Geometry: final body of the model. Coordinates: model frame, mm. Give positions to 0.01 mm unless a question says otherwise; leave off trailing zeros. Write each loop counter-clockwise with the first axis right and the second up, starting at its lowest first coordinate (ties: lowest second). Pieces come first, ordered by that corner, then holes. Notation, with made-up numbers: (-24, -16.5) - (4, -16.5) arc R20 cw to (4, 12.5) - close; hole circle Ø6 at (15, -3.75). An arc over 180 degrees is marked (long way). Use CSV: the item, a comma, the result in double quotes. Start each with the question number.
(1) First-contact query: pin 1 Ø1 at (y, z) = (5.5, -2) entering from -X; pin 2 Ø4 at (y, z) = (9, -1.5) entering from +X; pin 3 Ø1.5 at (y, z) = (26.5, 0.5) entering from -X. Flat tips, straight axial feed; report the tip coordinate or a pass-through.
(2) Section B-B on y = 13. Output: boundary loops of the cut face in (x, z), and give its area (3 significant figures).
(3) Section A-A on y = 3. Output: boundary loops of the cut face in (x, z), and give its area (3 significant figures).
(4) Line query: probe 1 along X at (y, z) = (14.5, -0.25); probe 2 along X at (y, z) = (8, -3); probe 3 along Y at (x, z) = (-3.5, 2.75). Output: solid intervals per line, ascending. Write a range as [from, to].
from build123d import *

# Parameters (mm, degrees)
EXTRUDE_1_DEPTH     = 4
CUT_EXTRUDE_1_DEPTH = 1.5
SKETCH_2_R          = 4
EXTRUDE_2_DEPTH     = 25
CUT_EXTRUDE_2_DEPTH = 5
CHAMFER_2_SIZE      = 1


with BuildPart() as part:
    # Эскиз1 → Бобышка-Вытянуть1 (new body, symmetric)
    with BuildSketch(Plane.XY):
        Polygon((8.9, 0), (-8.9, 0), (-8.9, 4), (-4, 4), (-4, 5.5), (4, 5.5), (4, 4), (8.9, 4), align=None)
    extrude(amount=EXTRUDE_1_DEPTH, both=True)

    # Эскиз3 → Вырез-Вытянуть1 (cut)
    with BuildSketch(Plane(origin=(0, 5.5, 0), x_dir=(1, 0, 0), z_dir=(0, 1, 0))):
        with BuildLine():
            Line((-4, 0), (-4, 4))
            Line((-4, 4), (0, 4))
            ThreePointArc((0, 4), (-2.828427125, 2.828427125), (-4, 0))
        make_face()
        with BuildLine():
            Line((0, -4), (4, -4))
            Line((4, -4), (4, 0))
            ThreePointArc((4, 0), (2.828427125, -2.828427125), (0, -4))
        make_face()
    extrude(amount=-CUT_EXTRUDE_1_DEPTH, mode=Mode.SUBTRACT)

    # Эскиз2 → Бобышка-Вытянуть2 (add)
    with BuildSketch(Plane(origin=(0, 5.5, 0), x_dir=(1, 0, 0), z_dir=(0, 1, 0))):
        with Locations(Location((0, 0, 0), (0, 0, 270))):  # turned: the seam where the file's is
            Circle(SKETCH_2_R)
    extrude(amount=EXTRUDE_2_DEPTH)

    # Эскиз4 → Вырез-Вытянуть2 (cut, through all)
    with BuildSketch(Plane(origin=(0, 4, 0), x_dir=(1, 0, 0), z_dir=(0, 1, 0))):
        with BuildLine():
            Line((-7.950471684, 4), (-8.9, 4))
            Line((-8.9, 4), (-8.9, 0))
            ThreePointArc((-8.9, 0), (-8.659364815, 2.055578022), (-7.950471684, 4))
        make_face()
        with BuildLine():
            Line((7.950471684, -4), (8.9, -4))
            Line((8.9, -4), (8.9, 0))
            ThreePointArc((8.9, 0), (8.659364815, -2.055578022), (7.950471684, -4))
        make_face()
    extrude(amount=-CUT_EXTRUDE_2_DEPTH, mode=Mode.SUBTRACT)

    # Вырез-По траектории1: sweep along a path in Эскиз6
    with BuildLine(Plane.XZ) as sweep_1_path:
        Line((0, -8.9), (8.9, -8.9))
        Line((8.9, -8.9), (8.9, 0))
        ThreePointArc((8.9, 0), (6.293250353, 6.293250353), (0, 8.9))
        Line((0, 8.9), (-8.9, 8.9))
        Line((-8.9, 8.9), (-8.9, 0))
        ThreePointArc((-8.9, 0), (-6.293250353, -6.293250353), (0, -8.9))
    # Эскиз5 → Вырез-По траектории1 (sweep, cut)
    with BuildSketch(Plane.XY.offset(4)):
        Polygon((-8.9, 2.5), (-4.8, 0), (-8.9, 0), align=None)
    sweep(path=sweep_1_path.line, transition=Transition.RIGHT, mode=Mode.SUBTRACT)

    # Фаска2
    chamfer_2_edges = [part.edges().sort_by_distance(p)[0] for p in [
        (0, 30.5, -4),
    ]]
    chamfer(chamfer_2_edges, length=CHAMFER_2_SIZE)


solid = part.part
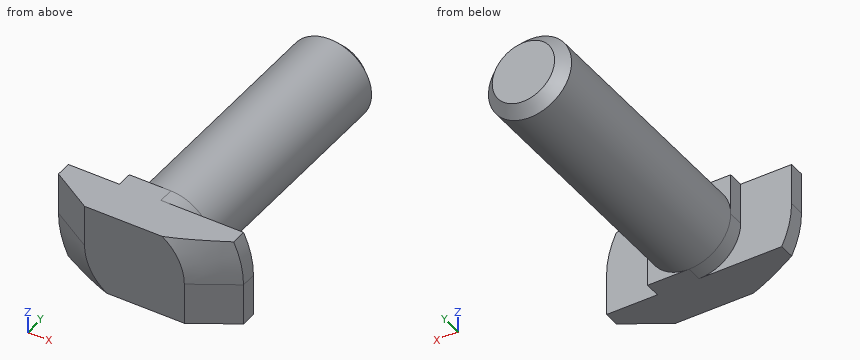
Check values:
1,pin 1,"stops at x = -3.71"
1,pin 2,"stops at x = 4"
1,pin 3,"stops at x = -4"
2,outline,"circle Ø8 at (0, 0)"
2,area,"50.3 mm²"
3,outline,"(-8.9, 0) arc R8.9 ccw to (-7.95, -4) - (8.9, -4) - (8.9, 0) arc R8.9 ccw to (7.95, 4) - (-8.9, 4) - close"
3,area,"140 mm²"
4,probe 1,"x = [-3.99, 3.99]"
4,probe 2,"x = [-2.65, 2.65]"
4,probe 3,"y = [0, 5.5]"
